```python
from build123d import *

# Parameters (mm, degrees)
F0_W     = 127
F0_H     = 76.2
F1_DEPTH = 38.1
F2_R     = 5.08
F4_DEPTH = 16.4
F6_DEPTH = 16.8


with BuildPart() as f1:
    # F0 (on Front) → F1 (new body)
    with BuildSketch(Plane.XZ):
        Rectangle(F0_W, F0_H)
    extrude(amount=F1_DEPTH)

    # F2
    f2_edges = [f1.edges().sort_by_distance(p)[0] for p in [
        (0, -38.1, 38.1),
        (0, 0, 38.1),
        (0, -38.1, -38.1),
        (0, 0, -38.1),
    ]]
    fillet(f2_edges, radius=F2_R)

    # F3 (on face) → F4 (cut)
    with BuildSketch(Plane.YZ.offset(63.5)):
        with BuildLine():
            Line((-28.02, 33.02), (-31.02, 33.02))
            ThreePointArc((-31.02, 33.02), (-32.434214, 32.434214), (-33.02, 31.02))
            Line((-33.02, 31.02), (-33.02, 18.22))
            ThreePointArc((-33.02, 18.22), (-32.434214, 16.805786), (-31.02, 16.22))
            Line((-31.02, 16.22), (-28.02, 16.22))
            ThreePointArc((-28.02, 16.22), (-26.605786, 16.805786), (-26.02, 18.22))
            Line((-26.02, 18.22), (-26.02, 31.02))
            ThreePointArc((-26.02, 31.02), (-26.605786, 32.434214), (-28.02, 33.02))
        make_face()
    extrude(amount=-F4_DEPTH, mode=Mode.SUBTRACT)

    # F5 (on face) → F6 (cut)
    with BuildSketch(Plane.YZ.offset(63.5)):
        with BuildLine():
            Line((-14.584209, 32.715682), (-17.584209, 32.715682))
            ThreePointArc((-17.584209, 32.715682), (-18.998423, 32.129895), (-19.584209, 30.715682))
            Line((-19.584209, 30.715682), (-19.584209, 17.915682))
            ThreePointArc((-19.584209, 17.915682), (-18.998423, 16.501468), (-17.584209, 15.915682))
            Line((-17.584209, 15.915682), (-14.584209, 15.915682))
            ThreePointArc((-14.584209, 15.915682), (-13.169996, 16.501468), (-12.584209, 17.915682))
            Line((-12.584209, 17.915682), (-12.584209, 30.715682))
            ThreePointArc((-12.584209, 30.715682), (-13.169996, 32.129895), (-14.584209, 32.715682))
        make_face()
    extrude(amount=-F6_DEPTH, mode=Mode.SUBTRACT)


solid = f1.part
```
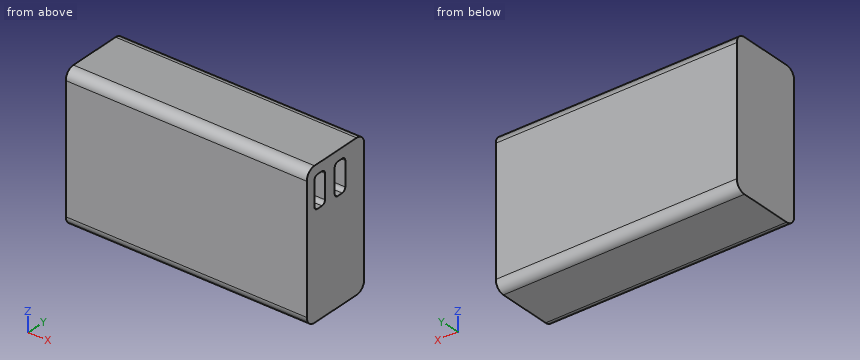
Part model, mm, in its own coordinate system. Give positions to 0.01 mm unless a question says otherwise; leave off trailing zeros. Write each loop counter-clockwise with the first axis right and the second up, starting at its lowest first coordinate (ties: lowest second). Pieces come first, ordered by that corner, then holes. Notation, with made-up numbers: (65.5, 79.25) -> (87.5, 79.25) arc R21 cw to (87.5, 104.25) -> close; hole circle Ø9 at (33.25, -36.5). An arc over 180 degrees is marked (long way). Put each result on its own line as item: value. Start each with the question number.
Item 1: Wall check: L1, parallel to Y at x = 48, z = 25.5; L2, parallel to X at y = -19, z = 20; L3, parallel to Z at x = -31.5, y = -34. Give the ranges that are in metal, low to high. Write a range as [from, to].
Item 2: Pin check, flat tips, straight feed: pin 1 Ø2 at (y, z) = (-14.5, 26) entering from +X; pin 2 Ø2 at (y, z) = (-30.5, 26.5) entering from +X. Stop position of each tip, or through.
Item 3: Cut at A-A (y = -16). List the corners of the cut face in (x, z), then the cut area to 3 significant figures.
Answer list:
1. L1: y = [-38.1, -33.02], [-26.02, -19.58], [-12.58, 0]
1. L2: x = [-63.5, 46.7]
1. L3: z = [-38, 38]
2. pin 1: stops at x = 46.7
2. pin 2: stops at x = 47.1
3. outline: (-63.5, -38.1) -> (63.5, -38.1) -> (63.5, 15.92) -> (46.7, 15.92) -> (46.7, 32.72) -> (63.5, 32.72) -> (63.5, 38.1) -> (-63.5, 38.1) -> close
3. area: 9,400 mm2
